For this review, use the dimensioned drawing (mm, ordinates from the lowest corner) and the shaded views. Give positions to 0.01 mm unless a question says otherwise; leave off trailing zeros. Write each loop counter-clockwise with the first axis right and the second up, starting at its lowest first coordinate (ties: lowest second). Pieces come first, ordered by that corner, then holes. Notation, with made-up numbers: M 12,80.25 L 37,80.25 A19 ccw 37,108.25 Z; hole C -31,54 d8. An arc over 180 degrees is marked long. Answer in a Markdown table with one row per item.
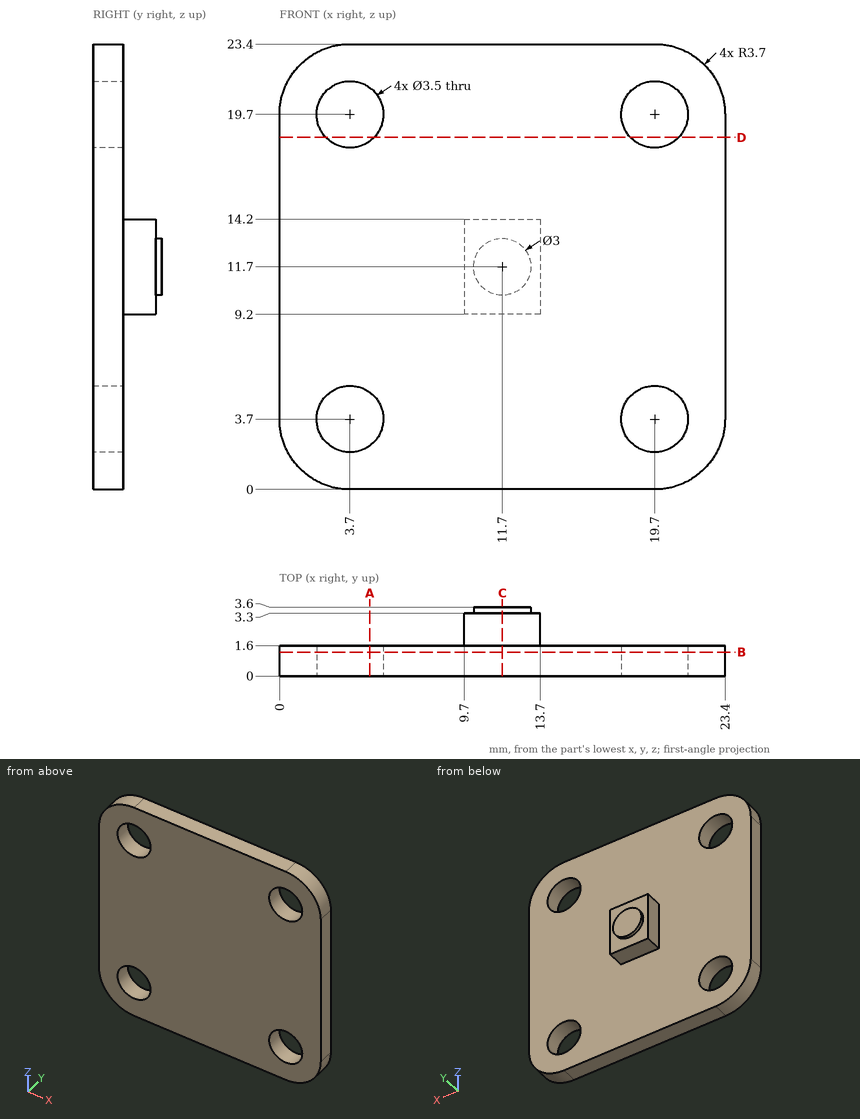
1) Add section D-D (z = 18.5). Write out the cut boundary in (x, y), and give its area (3 significant figures).
Geometry says:
| item | result |
|---|---|
| outline | M 0,0 L 2.43,0 L 2.43,1.6 L 0,1.6 Z; M 4.97,0 L 18.43,0 L 18.43,1.6 L 4.97,1.6 Z; M 20.97,0 L 23.4,0 L 23.4,1.6 L 20.97,1.6 Z |
| area | 29.3 mm^2 |
2) Add section A-A (x = 4.75). Write out the cut boundary in (y, z).
Geometry says:
| item | result |
|---|---|
| outline | M 0,0 L 1.6,0 L 1.6,2.3 L 0,2.3 Z; M 0,5.1 L 1.6,5.1 L 1.6,18.3 L 0,18.3 Z; M 0,21.1 L 1.6,21.1 L 1.6,23.4 L 0,23.4 Z |
3) Add section B-B (y = 1.25). Write out the cut boundary in (x, z), and give its area (3 significant figures).
Geometry says:
| item | result |
|---|---|
| outline | M 0,3.7 A3.7 ccw 3.7,0 L 19.7,0 A3.7 ccw 23.4,3.7 L 23.4,19.7 A3.7 ccw 19.7,23.4 L 3.7,23.4 A3.7 ccw 0,19.7 Z; hole C 3.7,3.7 d3.5; hole C 3.7,19.7 d3.5; hole C 19.7,3.7 d3.5; hole C 19.7,19.7 d3.5 |
| area | 497 mm^2 |
4) Insertion check: P1, Ø1.4, axis at y = 2.5, z = 12, coming from the +X side; P2, Ø3, axis at x = 3.7, z = 19.7, coming from the -Y side; P3, Ø2, axis at y = 0.5, z = 2.5, coming from the +X side; P4, Ø5, axis at x = 14.5, z = 6.5, coming from the +Y side. Each pin has a flat end and moves straight along its axis. Give the tip position at first contact, or say it passes through.
Geometry says:
| item | result |
|---|---|
| P1 | x = 13.7 |
| P2 | through |
| P3 | x = 23.39 |
| P4 | y = 1.6 |
5) To check wall thickness, follow probe 1 along X at (y, z) = (0.7, 19.7); probe 2 along X at (y, z) = (1.4, 4.75); probe 3 along Z at (x, y) = (4.5, 1.1). State the ranges of each line that lie inside material, in increasing order. Write a range as [from, to].
Geometry says:
| item | result |
|---|---|
| probe 1 | [0, 1.95], [5.45, 17.95], [21.45, 23.4] |
| probe 2 | [0, 2.3], [5.1, 18.3], [21.1, 23.4] |
| probe 3 | [0, 2.14], [5.26, 18.14], [21.26, 23.4] |
6) Add section C-C (x = 11.7). Write out the cut boundary in (y, z), and give its area (3 significant figures).
Geometry says:
| item | result |
|---|---|
| outline | M 0,0 L 1.6,0 L 1.6,9.2 L 3.3,9.2 L 3.3,10.2 L 3.6,10.2 L 3.6,13.2 L 3.3,13.2 L 3.3,14.2 L 1.6,14.2 L 1.6,23.4 L 0,23.4 Z |
| area | 46.8 mm^2 |
